from build123d import *

# Parameters (mm, degrees)
SKETCH_1_W                 = 125
SKETCH_1_H                 = 30
EXTRUDE_1_DEPTH            = 4
EXTRUDE_3_DEPTH            = 5
SKETCH_11_R                = 0.8
CUT_EXTRUDE_6_DEPTH        = 77.439518575
CUT_EXTRUDE_7_DEPTH        = 1.3
CUT_EXTRUDE_8_DEPTH        = 1.3
EXTRUDE_4_DEPTH            = 13
SKETCH_15_R                = 1.1
CUT_EXTRUDE_9_DEPTH        = 115.99682112
SKETCH_16_R                = 1.1
CUT_EXTRUDE_10_DEPTH       = 115.99682112
CUT_EXTRUDE_11_DEPTH       = 66.576291447
CUT_EXTRUDE_11_DEPTH_BACK  = 66.576291447
SKETCH_17_R                = 1.1
SKETCH_17_R_2              = 2.6
CUT_EXTRUDE_START          = -2
CUT_EXTRUDE_12_OUTLINE_R   = 2.2
CUT_EXTRUDE_12_OUTLINE_R_2 = 1.1
CUT_EXTRUDE_12_DEPTH       = 9.65934245
SKETCH_19_R                = 1.6
CUT_EXTRUDE_13_DEPTH       = 66.576291447


# Read off the part's stored shape, not the designer's step: the extrude step
with BuildPart() as part:
    # Sketch 1 → Extrude 1 (new body)
    with BuildSketch(Plane(origin=(0, 0, 0), x_dir=(1, 0, 0), z_dir=(0, 1, 0))):
        Rectangle(SKETCH_1_W, SKETCH_1_H)
    extrude(amount=EXTRUDE_1_DEPTH)

    # Sketch 4 → Extrude 3 (add)
    with BuildSketch(Plane.XY.offset(7)):
        with BuildLine():
            Line((-4, 15), (-4, 17))
            Line((-4, 17), (-10.5, 17))
            Line((-10.5, 17), (-10.5, 4))
            Line((-10.5, 4), (-7.375, 4))
            Line((-7.375, 4), (-7.375, 9.8))
            Line((-7.375, 9.8), (-4.775, 9.8))
            Line((-4.775, 9.8), (-4.775, 4))
            Line((-4.775, 4), (4.775, 4))
            Line((4.775, 4), (4.775, 9.8))
            Line((4.775, 9.8), (7.375, 9.8))
            Line((7.375, 9.8), (7.375, 4))
            Line((7.375, 4), (10.5, 4))
            Line((10.5, 4), (10.5, 17))
            Line((10.5, 17), (4, 17))
            Line((4, 17), (4, 15))
            ThreePointArc((4, 15), (0, 11), (-4, 15))
        make_face()
    extrude(amount=-EXTRUDE_3_DEPTH)

    # Sketch 11 → Cut-Extrude 6 (cut, through all)
    with BuildSketch(Plane(origin=(10.5, 0, 0), x_dir=(0, 0, -1), z_dir=(1, 0, 0))):
        with Locations((-4.6, 6.6)):
            Circle(SKETCH_11_R)
    extrude(amount=-CUT_EXTRUDE_6_DEPTH, mode=Mode.SUBTRACT)

    # Sketch 12 → Cut-Extrude 7 (cut)
    with BuildSketch(Plane.ZY.offset(3.775)):
        Polygon((5.466025404, 9.1), (7, 9.1), (7, 4.1), (5.466025404, 4.1), (3.156624327, 4.1), (1.713248654, 6.6), (3.156624327, 9.1), align=None)
    extrude(amount=-CUT_EXTRUDE_7_DEPTH, mode=Mode.SUBTRACT)

    # Sketch 13 → Cut-Extrude 8 (cut)
    with BuildSketch(Plane(origin=(3.775, 0, 0), x_dir=(0, 0, -1), z_dir=(1, 0, 0))):
        Polygon((-5.466025404, 9.1), (-7, 9.1), (-7, 4.1), (-5.466025404, 4.1), (-3.156624327, 4.1), (-1.713248654, 6.6), (-3.156624327, 9.1), align=None)
    extrude(amount=-CUT_EXTRUDE_8_DEPTH, mode=Mode.SUBTRACT)

    # Sketch 14 → Extrude 4 (add)
    with BuildSketch(Plane(origin=(0, 4, 0), x_dir=(1, 0, 0), z_dir=(0, 1, 0))):
        Polygon((55, -2), (52.5, 2.330127019), (55.964101615, 4.330127019), (58.464101615, 0), align=None)
        Polygon((49.3, 7.872689603), (46.8, 12.202816622), (50.264101615, 14.202816622), (52.764101615, 9.872689603), align=None)
        Polygon((-55, -2), (-52.5, 2.330127019), (-55.964101615, 4.330127019), (-58.464101615, 0), align=None)
        Polygon((-49.3, 7.872689603), (-46.8, 12.202816622), (-50.264101615, 14.202816622), (-52.764101615, 9.872689603), align=None)
    extrude(amount=EXTRUDE_4_DEPTH)

    # Sketch 15 → Cut-Extrude 9 (cut, through all)
    with BuildSketch(Plane(origin=(-43.848076211, 0, -25.315698604), x_dir=(-0.5000000000000007, 0, 0.8660254037844383), z_dir=(-0.8660254037844383, 0, -0.5000000000000007))):
        with Locations((15.332050808, 14.2)):
            Circle(SKETCH_15_R)
        with Locations((26.732050808, 14.2)):
            Circle(SKETCH_15_R)
    extrude(amount=-CUT_EXTRUDE_9_DEPTH, mode=Mode.SUBTRACT)

    # Sketch 16 → Cut-Extrude 10 (cut, through all)
    with BuildSketch(Plane(origin=(43.848076211, 0, -25.315698604), x_dir=(-0.5000000000000019, 0, -0.8660254037844377), z_dir=(0.8660254037844377, 0, -0.5000000000000019))):
        with Locations((-26.732050808, 14.2)):
            Circle(SKETCH_16_R)
        with Locations((-15.332050808, 14.2)):
            Circle(SKETCH_16_R)
    extrude(amount=-CUT_EXTRUDE_10_DEPTH, mode=Mode.SUBTRACT)

    # Sketch 17 → Cut-Extrude 11 (cut, two sides: drawn at the far end of the back side and taken through both)
    with BuildSketch(Plane(origin=(0, 4, 0), x_dir=(1, 0, 0), z_dir=(0, 1, 0)).offset(-CUT_EXTRUDE_11_DEPTH_BACK)):
        with Locations(Location((-14.4, 0, 0), (0, 0, 270))):
            Circle(SKETCH_17_R)
        with Locations(Location((17, 0, 0), (0, 0, 270))):
            Circle(SKETCH_17_R)
        with Locations(Location((0, 6.4, 0), (0, 0, 270))):
            Circle(SKETCH_17_R)
        with Locations(Location((0, -6.4, 0), (0, 0, 270))):
            Circle(SKETCH_17_R)
        with Locations(Location((0, 0, 0), (0, 0, 270))):
            Circle(SKETCH_17_R_2)
    extrude(amount=CUT_EXTRUDE_11_DEPTH + CUT_EXTRUDE_11_DEPTH_BACK, mode=Mode.SUBTRACT)

    # Cut-Extrude 12 outline → Cut-Extrude 12 (cut)
    # profile 1 of 4: a face of its own
    with BuildSketch(Plane(origin=(0, 4, 0), x_dir=(1, 0, 0), z_dir=(0, 1, 0)).offset(CUT_EXTRUDE_START)):
        with Locations((-14.4, 0)):
            Circle(CUT_EXTRUDE_12_OUTLINE_R)
        with Locations((-14.4, 0)):
            Circle(CUT_EXTRUDE_12_OUTLINE_R_2, mode=Mode.SUBTRACT)
    # profile 2 of 4: a face of its own
    with BuildSketch(Plane(origin=(0, 4, 0), x_dir=(1, 0, 0), z_dir=(0, 1, 0)).offset(CUT_EXTRUDE_START)):
        with Locations((17, 0)):
            Circle(CUT_EXTRUDE_12_OUTLINE_R)
        with Locations((17, 0)):
            Circle(CUT_EXTRUDE_12_OUTLINE_R_2, mode=Mode.SUBTRACT)
    # profile 3 of 4: a face of its own
    with BuildSketch(Plane(origin=(0, 4, 0), x_dir=(1, 0, 0), z_dir=(0, 1, 0)).offset(CUT_EXTRUDE_START)):
        with Locations((0, -6.4)):
            Circle(CUT_EXTRUDE_12_OUTLINE_R)
        with Locations((0, -6.4)):
            Circle(CUT_EXTRUDE_12_OUTLINE_R_2, mode=Mode.SUBTRACT)
    # profile 4 of 4: a face of its own
    with BuildSketch(Plane(origin=(0, 4, 0), x_dir=(1, 0, 0), z_dir=(0, 1, 0)).offset(CUT_EXTRUDE_START)):
        with Locations((0, 6.4)):
            Circle(CUT_EXTRUDE_12_OUTLINE_R)
        with Locations((0, 6.4)):
            Circle(CUT_EXTRUDE_12_OUTLINE_R_2, mode=Mode.SUBTRACT)
    extrude(amount=CUT_EXTRUDE_12_DEPTH, mode=Mode.SUBTRACT)

    # Sketch 19 → Cut-Extrude 13 (cut, through all)
    with BuildSketch(Plane(origin=(0, 4, 0), x_dir=(1, 0, 0), z_dir=(0, 1, 0))):
        with Locations(Location((-57.5, -10, 0), (0, 0, 270))):
            Circle(SKETCH_19_R)
        with Locations(Location((57.5, -10, 0), (0, 0, 270))):
            Circle(SKETCH_19_R)
    extrude(amount=-CUT_EXTRUDE_13_DEPTH, mode=Mode.SUBTRACT)


solid = part.part
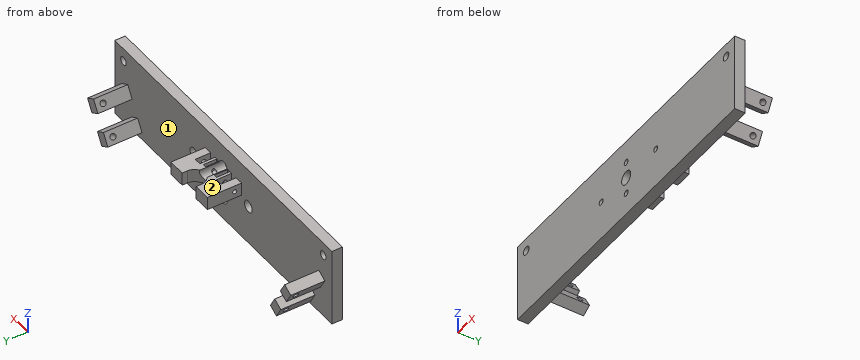
Model file for the job. Use its own axes, mm. Face numbers are marked on the shaded views. Round coordinates to 2 decimals unless told otherwise and drop trailing zeros. Loops run counter-clockwise (first coordinate to the right, second up) from the corner with the lowest first, then second, coordinate; pieces in that order, holes last. Notation, with made-up numbers: M 24.5,29 L 31.5,29 A30 cw 31.5,63 Z; hole C -24,11.25 d5. An arc over 180 degrees is marked long. One line per question, with ' | ' between items.
1) Band-saw the part on B-B (x = -37.5). Give the cut face in (y, z).
Solved:
outline: M 0,-15 L 4,-15 L 4,15 L 0,15 Z
2) Band-saw the part on C-C (z = 13.25). Give the cut face in (x, y), then the cut area to 3 significant figures.
Solved:
outline: M -62.5,0 L 62.5,0 L 62.5,4 L -62.5,4 Z | area: 500 mm²
3) Mould opens along X. For the marked faces 1 and 2 say: +X half, -X half, draft (parallel to the pull), parting line (faces both ways), or undercut.
Solved:
face 1: undercut | face 2: draft
4) Flat gauge pins, fed straight in: pin 1 (3 mm diameter, centred on x = 38, z = 7, fed in from -Y); pin 2 (3.5 mm diameter, centred on x = 0, z = 6.4, fed in from +Y); pin 3 (6 mm diameter, centred on x = -40.5, z = -11, fed in from +Y); pin 4 (1 mm diameter, centred on y = 15, z = -10.5, fed in from +X). Where does each tip first touch, or does it go through?
Solved:
pin 1: stops at y = 0 | pin 2: stops at y = 2 | pin 3: stops at y = 4 | pin 4: stops at x = 52.69
5) Band-saw the part on A-A (z = -6.4). Give the cut face in (x, y).
Solved:
outline: M -62.5,0 L -1.1,0 L -1.1,2 L -2.2,2 L -2.2,4 L -62.5,4 Z; M 1.1,0 L 62.5,0 L 62.5,4 L 2.2,4 L 2.2,2 L 1.1,2 Z
6) Drill centre lines: line 1 along X through (y, z) = (1.4, 0); line 2 along X through (y, z) = (8.25, 2.75) (3 decimals); line 3 along Z through (x, y) = (0, 1.1). Where is each one in solid material? Low to high.
Solved:
line 1: x = -62.5 to -15.5, -13.3 to -2.6, 2.6 to 15.9, 18.1 to 62.5 | line 2: x = -10.5 to -7.375, -4.775 to -3.775, -2.475 to 2.475, 3.775 to 4.775, 7.375 to 10.5 | line 3: z = -15 to -7.5, -5.3 to -2.6, 2.6 to 5.3, 7.5 to 15
